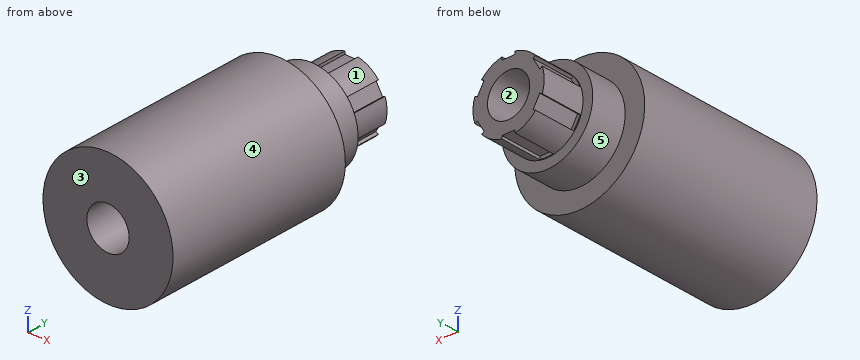
```python
from build123d import *

# Parameters (mm, degrees)
F3_DEPTH = 17.1


with BuildPart() as f1:
    # F0 (on Right) → F1 (revolve)
    with BuildSketch(Plane.YZ):
        Polygon((17.869576, 26.562618), (-59.984905, 26.562618), (-59.984905, 8.62), (50, 8.62), (50, 14.562618), (32.493035, 14.562618), (32.493035, 18.562618), (17.869576, 18.562618), align=None)
    revolve(axis=Axis((0, 1.113363, 0), (0, 1, 0)))


with BuildPart() as f3:
    # F2 (on face) → F3 (new body)
    with BuildSketch(Plane(origin=(0, 50, 0), x_dir=(-1, 0, 0), z_dir=(0, 1, 0))):
        with BuildLine():
            Line((-2.716261, 14.562618), (-2.716261, 14.307053))
            ThreePointArc((-2.716261, 14.307053), (-1.364129, 14.498586), (0, 14.562618))
            Line((0, 14.562618), (-2.716261, 14.562618))
        make_face()
        with BuildLine():
            Line((2.716261, 14.562618), (0, 14.562618))
            ThreePointArc((0, 14.562618), (1.364129, 14.498586), (2.716261, 14.307053))
            Line((2.716261, 14.307053), (2.716261, 14.562618))
        make_face()
        with BuildLine():
            ThreePointArc((-12.611597, 7.281309), (-11.87408, 8.430663), (-11.032141, 9.505878))
            Line((-11.032141, 9.505878), (-11.253467, 9.63366))
            Line((-11.253467, 9.63366), (-12.611597, 7.281309))
        make_face()
        with BuildLine():
            ThreePointArc((-13.748402, 4.801175), (-13.238208, 6.067923), (-12.611597, 7.281309))
            Line((-12.611597, 7.281309), (-13.969728, 4.928958))
            Line((-13.969728, 4.928958), (-13.748402, 4.801175))
        make_face()
        with BuildLine():
            ThreePointArc((-12.611597, -7.281309), (-13.238208, -6.067923), (-13.748402, -4.801175))
            Line((-13.748402, -4.801175), (-13.969728, -4.928958))
            Line((-13.969728, -4.928958), (-12.611597, -7.281309))
        make_face()
        with BuildLine():
            ThreePointArc((-11.032141, -9.505878), (-11.87408, -8.430663), (-12.611597, -7.281309))
            Line((-12.611597, -7.281309), (-11.253467, -9.63366))
            Line((-11.253467, -9.63366), (-11.032141, -9.505878))
        make_face()
        with BuildLine():
            ThreePointArc((0, -14.562618), (-1.364129, -14.498586), (-2.716261, -14.307053))
            Line((-2.716261, -14.307053), (-2.716261, -14.562618))
            Line((-2.716261, -14.562618), (0, -14.562618))
        make_face()
        with BuildLine():
            ThreePointArc((2.716261, -14.307053), (1.364129, -14.498586), (0, -14.562618))
            Line((0, -14.562618), (2.716261, -14.562618))
            Line((2.716261, -14.562618), (2.716261, -14.307053))
        make_face()
        with BuildLine():
            Line((11.253467, -9.63366), (12.611597, -7.281309))
            ThreePointArc((12.611597, -7.281309), (11.87408, -8.430663), (11.032141, -9.505878))
            Line((11.032141, -9.505878), (11.253467, -9.63366))
        make_face()
        with BuildLine():
            Line((13.969728, -4.928958), (13.748402, -4.801175))
            ThreePointArc((13.748402, -4.801175), (13.238208, -6.067923), (12.611597, -7.281309))
            Line((12.611597, -7.281309), (13.969728, -4.928958))
        make_face()
        with BuildLine():
            Line((13.969728, 4.928958), (12.611597, 7.281309))
            ThreePointArc((12.611597, 7.281309), (13.238208, 6.067923), (13.748402, 4.801175))
            Line((13.748402, 4.801175), (13.969728, 4.928958))
        make_face()
        with BuildLine():
            Line((11.253467, 9.63366), (11.032141, 9.505878))
            ThreePointArc((11.032141, 9.505878), (11.87408, 8.430663), (12.611597, 7.281309))
            Line((12.611597, 7.281309), (11.253467, 9.63366))
        make_face()
        with BuildLine():
            Line((-2.716261, 14.307053), (-2.716261, 13.132972))
            Line((-2.716261, 13.132972), (2.716261, 13.132972))
            Line((2.716261, 13.132972), (2.716261, 14.307053))
            ThreePointArc((2.716261, 14.307053), (1.364129, 14.498586), (0, 14.562618))
            ThreePointArc((0, 14.562618), (-1.364129, 14.498586), (-2.716261, 14.307053))
        make_face()
        with BuildLine():
            Line((-12.731618, -4.214135), (-13.748402, -4.801175))
            ThreePointArc((-13.748402, -4.801175), (-13.238208, -6.067923), (-12.611597, -7.281309))
            ThreePointArc((-12.611597, -7.281309), (-11.87408, -8.430663), (-11.032141, -9.505878))
            Line((-11.032141, -9.505878), (-10.015357, -8.918837))
            Line((-10.015357, -8.918837), (-12.731618, -4.214135))
        make_face()
        with BuildLine():
            Line((-2.716261, -13.132972), (-2.716261, -14.307053))
            ThreePointArc((-2.716261, -14.307053), (-1.364129, -14.498586), (0, -14.562618))
            ThreePointArc((0, -14.562618), (1.364129, -14.498586), (2.716261, -14.307053))
            Line((2.716261, -14.307053), (2.716261, -13.132972))
            Line((2.716261, -13.132972), (-2.716261, -13.132972))
        make_face()
        with BuildLine():
            ThreePointArc((12.611597, -7.281309), (13.238208, -6.067923), (13.748402, -4.801175))
            Line((13.748402, -4.801175), (12.731618, -4.214135))
            Line((12.731618, -4.214135), (10.015357, -8.918837))
            Line((10.015357, -8.918837), (11.032141, -9.505878))
            ThreePointArc((11.032141, -9.505878), (11.87408, -8.430663), (12.611597, -7.281309))
        make_face()
        with BuildLine():
            ThreePointArc((12.611597, 7.281309), (11.87408, 8.430663), (11.032141, 9.505878))
            Line((11.032141, 9.505878), (10.015357, 8.918837))
            Line((10.015357, 8.918837), (12.731618, 4.214135))
            Line((12.731618, 4.214135), (13.748402, 4.801175))
            ThreePointArc((13.748402, 4.801175), (13.238208, 6.067923), (12.611597, 7.281309))
        make_face()
        with BuildLine():
            Line((-10.015357, 8.918837), (-11.032141, 9.505878))
            ThreePointArc((-11.032141, 9.505878), (-11.87408, 8.430663), (-12.611597, 7.281309))
            ThreePointArc((-12.611597, 7.281309), (-13.238208, 6.067923), (-13.748402, 4.801175))
            Line((-13.748402, 4.801175), (-12.731618, 4.214135))
            Line((-12.731618, 4.214135), (-10.015357, 8.918837))
        make_face()
    extrude(amount=-F3_DEPTH)


with BuildPart() as f1_1:
    add(f1.part)

    # F4: cut F3
    add(f3.part, mode=Mode.SUBTRACT)


solid = f1_1.part
```
Read the model definition and answer for the solid it produces. Units are mm, in the model's axes. Face numbers are marked on the shaded views. A direction names the side the tool comes from. Coordinates: 2 decimals unless noted, no trailing zeros. Write each loop counter-clockwise with the first axis right and the second up, starting at its lowest first coordinate (ties: lowest second). Pieces come first, ordered by that corner, then holes. Notation, with made-up numbers: (-18.5, 77) -> (10.5, 77) arc R14 cw to (10.5, 90) -> close; hole circle Ø6 at (57, 61.5). An arc over 180 degrees is marked (long way). Answer as a JSON object with one key per item and string values.
Q1. The part is cut by section D-D on y = 23. Give the vertices of the cut face in (x, z), then the cut area to 3 significant figures.
The answers:
{"outline": "circle Ø37.13 at (0, 0); hole circle Ø17.24 at (0, 0)", "area": "849 mm2"}
Q2. Consider line 1 (X direction, y = -17, z = 0); line 2 (Y direction, x = 18.5, z = 14); line 3 (Z direction, x = 6.5, y = 9.5). Determine where each line is inside the solid, lowest interval first. Write a range as [from, to].
The answers:
{"line 1": "x = [-26.56, -8.62], [8.62, 26.56]", "line 2": "y = [-59.98, 17.87]", "line 3": "z = [-25.76, -5.66], [5.66, 25.76]"}
Q3. The part is cut by section B-B on z = 0. Give the vertices of the cut face in (x, y), then the cut area to 3 significant figures.
The answers:
{"outline": "(-26.56, -59.98) -> (-8.62, -59.98) -> (-8.62, 50) -> (-14.56, 50) -> (-14.56, 32.49) -> (-18.56, 32.49) -> (-18.56, 17.87) -> (-26.56, 17.87) -> close; (8.62, -59.98) -> (26.56, -59.98) -> (26.56, 17.87) -> (18.56, 17.87) -> (18.56, 32.49) -> (14.56, 32.49) -> (14.56, 50) -> (8.62, 50) -> close", "area": "3,290 mm2"}
Q4. The part is cut by section A-A on x = 0. Give the vertices of the cut face in (y, z).
The answers:
{"outline": "(-59.98, -26.56) -> (17.87, -26.56) -> (17.87, -18.56) -> (32.49, -18.56) -> (32.49, -14.56) -> (32.9, -14.56) -> (32.9, -13.13) -> (50, -13.13) -> (50, -8.62) -> (-59.98, -8.62) -> close; (-59.98, 8.62) -> (50, 8.62) -> (50, 13.13) -> (32.9, 13.13) -> (32.9, 14.56) -> (32.49, 14.56) -> (32.49, 18.56) -> (17.87, 18.56) -> (17.87, 26.56) -> (-59.98, 26.56) -> close"}
Q5. Determine the mould class of the marked faces 1, 2 and 3 for opening direction Z: pulls with the +Z half, pulls with the -Z half, needs draft (parallel to the pull), parting line crosses it, or undercut.
The answers:
{"face 1": "parting line crosses it", "face 2": "undercut", "face 3": "needs draft"}
Q6. Flat-ended cylindrical pins translate along their axes: pin 1 Ø1 at (x, y) = (-1, 28.5) entering from +Z; pin 2 Ø8 at (y, z) = (7, -2.5) entering from -X; pin 3 Ø1.3 at (y, z) = (42.5, -14) entering from +X. Find the tip coordinate at first contact, or state that the pin passes through.
The answers:
{"pin 1": "stops at z = 18.56", "pin 2": "stops at x = -26.56", "pin 3": "stops at x = 5.82"}
Q7. A tool of negligible diameter and unlimited length cuts with its end or side. For the marked faces 4 and 5, from which of +Z, -Z, +X, -X, +Y, -Y can it reach the whole face along a straight path? Write none if from no direction.
The answers:
{"face 4": "+Y, -Y", "face 5": "+Y"}
Q8. The part is cut by section C-C on x = -7.5. Give the vertices of the cut face in (y, z), then the cut area to 3 significant figures.
The answers:
{"outline": "(-59.98, -25.48) -> (17.87, -25.48) -> (17.87, -16.98) -> (32.49, -16.98) -> (32.49, -12.48) -> (50, -12.48) -> (50, -4.25) -> (-59.98, -4.25) -> close; (-59.98, 4.25) -> (50, 4.25) -> (50, 12.48) -> (32.49, 12.48) -> (32.49, 16.98) -> (17.87, 16.98) -> (17.87, 25.48) -> (-59.98, 25.48) -> close", "area": "3,970 mm2"}
